Check sheet for the modelled part. Datum: model origin and axes. Units: mm. A direction names the side the tool comes from. Give positions to 0.01 mm unless a question says otherwise; leave off trailing zeros. Order: outer loops, then holes, each group sorted by start corner. A loop starts at its lowest first (then second) coordinate and runs counter-clockwise, first axis right, second up. Notation, with made-up numbers: (30.25, 79.25) -> (60.25, 79.25) arc R32 cw to (60.25, 105.25) -> close; hole circle Ø10 at (3.5, 83). An arc over 180 degrees is marked (long way). Answer in a Markdown table with one row per item. Add a question column.
(1) Cross-section at C-C (x = 17). Record the cut outline in (y, z), then the cut area to 3 significant figures.
(2) Thickness scan on L1, parallel to X at y = 48.5, z = 11.5; L2, parallel to Y at x = 26, z = 42; L3, parallel to X at y = 19, z = 58. Record the ranges inside material, lowest first. Write a range as [from, to].
(3) Cross-section at B-B (y = 49.5). Record the cut outline in (x, z).
(4) Set-up check for faces 4 (the face through (2, 84, 60)), 5 (the face through (49, 51, 41)), 6 (the face through (0, 51, 38)): record each of +Z, -Z, +X, -X, +Y, -Y from which the full face is reachable in a straight line by a thin tool's end or side.
(5) Cross-section at D-D (z = 48). Record the cut outline in (x, y), then the cut area to 3 significant figures.
(6) Release check for a two-part mould opening along X. For faces 1 (the face through (26, 102, 41)), 2 (the face through (25, 53, 0)), 3 (the face through (2, 21, 23)) record: released by +X, released by -X, zero draft, split by the parting line, or undercut.
(7) Go/stop test with a flat-tipped pin: pin 1 (4 mm diameter, centred on x = 43, y = 61, fed in from +Z). Record where the tip stops, or that it passes through.
(8) Cross-section at A-A (z = 22). Record the cut outline in (x, y), then the cut area to 3 significant figures.
```python
from build123d import *

# Parameters (mm, degrees)
SKETCH_W        = 51
SKETCH_H        = 104
PAD_DEPTH       = 78
SKETCH001_W     = 45
SKETCH001_H     = 100
POCKET_DEPTH    = 75
FILLET_R        = 1
SKETCH002_W     = 20.5
SKETCH002_H     = 6.5
POCKET001_DEPTH = 2


with BuildPart() as part:
    # Sketch → Pad (new body)
    with BuildSketch(Plane.XY):
        with Locations((25.5, 52)):
            Rectangle(SKETCH_W, SKETCH_H)
    extrude(amount=PAD_DEPTH)

    # Sketch001 (on Face6 of Pad) → Pocket (cut)
    with BuildSketch(Plane.XY.offset(78)):
        with Locations((26.5, 52)):
            Rectangle(SKETCH001_W, SKETCH001_H)
    extrude(amount=-POCKET_DEPTH, mode=Mode.SUBTRACT)

    # Fillet
    fillet_edges = [part.edges().sort_by_distance(p)[0] for p in [
        (51, 0, 39),
        (51, 104, 39),
        (51, 52, 0),
        (25.5, 0, 0),
        (51, 52, 78),
        (25.5, 0, 78),
        (25.5, 104, 78),
        (25.5, 104, 0),
    ]]
    fillet(fillet_edges, radius=FILLET_R)

    # Sketch002 (on Face2 of Fillet) → Pocket001 (cut, symmetric)
    with BuildSketch(Plane(origin=(0, 0, 0), x_dir=(0, -1, 0), z_dir=(-1, 0, 0))):
        with Locations((-84.25, 59.75)):
            Rectangle(SKETCH002_W, SKETCH002_H)
        with Locations((-84.25, 23.25)):
            Rectangle(SKETCH002_W, SKETCH002_H)
        with Locations((-21.25, 59.75)):
            Rectangle(SKETCH002_W, SKETCH002_H)
        with Locations((-21.25, 23.25)):
            Rectangle(SKETCH002_W, SKETCH002_H)
        with Locations((-53.276467, 59.75)):
            Rectangle(SKETCH002_W, SKETCH002_H)
        with Locations((-52.75, 23.25)):
            Rectangle(SKETCH002_W, SKETCH002_H)
    extrude(amount=POCKET001_DEPTH, both=True, mode=Mode.SUBTRACT)


solid = part.part
```
Answer below:
| question | item | result |
|---|---|---|
| 1 | outline | (0, 1) arc R1 ccw to (1, 0) -> (103, 0) arc R1 ccw to (104, 1) -> (104, 77) arc R1 ccw to (103, 78) -> (102, 78) -> (102, 3) -> (2, 3) -> (2, 78) -> (1, 78) arc R1 ccw to (0, 77) -> close |
| 1 | area | 611 mm² |
| 2 | L1 | x = [0, 4], [49, 51] |
| 2 | L2 | y = [0, 2], [102, 104] |
| 2 | L3 | x = [2, 4], [49, 51] |
| 3 | outline | (0, 0) -> (50, 0) arc R1 ccw to (51, 1) -> (51, 77) arc R1 ccw to (50, 78) -> (49, 78) -> (49, 3) -> (4, 3) -> (4, 78) -> (0, 78) -> (0, 63) -> (2, 63) -> (2, 56.5) -> (0, 56.5) -> (0, 26.5) -> (2, 26.5) -> (2, 20) -> (0, 20) -> close |
| 4 | face 4 | -X |
| 4 | face 5 | +Z |
| 4 | face 6 | +Z, -Z, -X, +Y, -Y |
| 5 | outline | (0, 0) -> (50, 0) arc R1 ccw to (51, 1) -> (51, 103) arc R1 ccw to (50, 104) -> (0, 104) -> close; hole (4, 2) -> (49, 2) -> (49, 102) -> (4, 102) -> close |
| 5 | area | 804 mm² |
| 6 | face 1 | undercut |
| 6 | face 2 | zero draft |
| 6 | face 3 | released by -X |
| 7 | pin 1 | stops at z = 3 |
| 8 | outline | (0, 0) -> (50, 0) arc R1 ccw to (51, 1) -> (51, 103) arc R1 ccw to (50, 104) -> (0, 104) -> (0, 94.5) -> (2, 94.5) -> (2, 74) -> (0, 74) -> (0, 63) -> (2, 63) -> (2, 42.5) -> (0, 42.5) -> (0, 31.5) -> (2, 31.5) -> (2, 11) -> (0, 11) -> close; hole (4, 2) -> (49, 2) -> (49, 102) -> (4, 102) -> close |
| 8 | area | 681 mm² |
